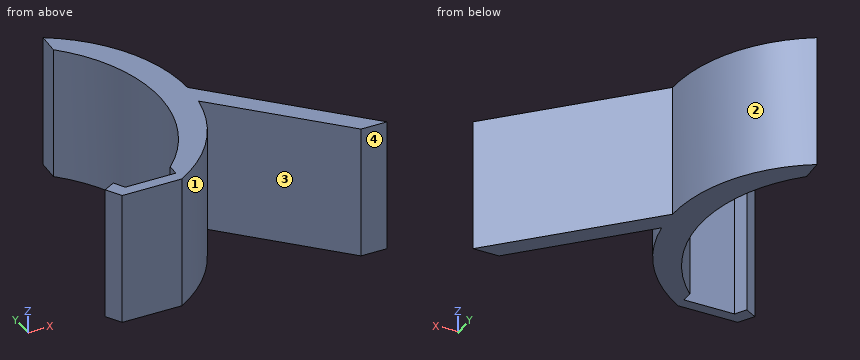
```python
from build123d import *

# Parameters (mm, degrees)
F1_DEPTH = 76.2


with BuildPart() as f1:
    # F0 (on Top) → F1 (new body)
    with BuildSketch(Plane.XY):
        Polygon((-34.220355, 0), (-25.4, 0), (-29.066174, 6.35), (-32.732348, 12.7), (-39.347615, 8.880674), align=None)
        with BuildLine():
            Line((-25.4, 0), (0, 0))
            ThreePointArc((0, 0), (27.857567, 26.408715), (41.984283, 62.100452))
            ThreePointArc((41.984283, 62.100452), (42.827748, 69.127812), (43.109499, 76.2))
            ThreePointArc((43.109499, 76.2), (31.585159, 119.974618), (0, 152.4))
            Line((0, 152.4), (-0.635, 139.7))
            ThreePointArc((-0.635, 139.7), (26.365937, 76.333417), (0, 12.7))
            Line((0, 12.7), (0, 6.35))
            Line((0, 6.35), (-29.066174, 6.35))
            Line((-29.066174, 6.35), (-25.4, 0))
        make_face()
        with BuildLine():
            ThreePointArc((43.109499, 76.2), (42.827748, 69.127812), (41.984283, 62.100452))
            Line((41.984283, 62.100452), (102.847256, 0))
            Line((102.847256, 0), (117.791057, 0))
            Line((117.791057, 0), (43.109499, 76.2))
        make_face()
    extrude(amount=F1_DEPTH)


solid = f1.part
```
Here's how the part is built. I have some questions about the finished solid (model axes, mm). Face numbers are marked on the shaded views. Coordinates: 2 decimals unless noted, no trailing zeros. Write each loop counter-clockwise with the first axis right and the second up, starting at its lowest first coordinate (ties: lowest second). Pieces come first, ordered by that corner, then holes. Notation, with made-up numbers: (88.5, 72) -> (138.5, 72) arc R31 ccw to (138.5, 102) -> close; hole circle Ø8 at (65.25, -25.5). An arc over 180 degrees is marked (long way). Use a Markdown table: item, result. Add a question column.
(1) We'd pull the mould along X, two halves only. Please class the marked faces 1, 2, 3 and 4: +X half, -X half, draft (parallel to the pull), parting line (faces both ways), or undercut.
(2) If we section it at D-D, the plane x = -20.5: Write out the boundary of the cut face in (y, z), and give its area (3 significant figures).
(3) I'm going to push flat-ended pins straight in: P1, Ø14.5, axis at x = -20.5, z = 48.5, coming from the +Y side; P2, Ø4, axis at y = 136.5, z = 45.5, coming from the -X side; P3, Ø10, axis at y = 75, z = 33.5, coming from the -X side. Where does each tip first touch, or does it pass through?
(4) If we section it at B-B, the plane y = 24.5: Write out the boundary of the cut face in (x, z).
(5) If we section it at C-C, the plane x = 22.5: Write out the boundary of the cut face in (y, z), and give its area (3 significant figures).
(6) Please list where these lines run through material, in increasing order: line 1 (X direction, y = 12.5, z = 72); line 2 (Y direction, x = -9, z = 60); line 3 (X direction, y = 17.5, z = 10.5).
Outcome:
| question | item | result |
|---|---|---|
| 1 | face 1 | undercut |
| 1 | face 2 | +X half |
| 1 | face 3 | undercut |
| 1 | face 4 | draft |
| 2 | outline | (0, 0) -> (6.35, 0) -> (6.35, 76.2) -> (0, 76.2) -> close |
| 2 | area | 484 mm^2 |
| 3 | P1 | stops at y = 6.35 |
| 3 | P2 | stops at x = 0.58 |
| 3 | P3 | stops at x = 26.17 |
| 4 | outline | (10.01, 0) -> (26.53, 0) -> (26.53, 76.2) -> (10.01, 76.2) -> close; (78.84, 0) -> (93.78, 0) -> (93.78, 76.2) -> (78.84, 76.2) -> close |
| 5 | outline | (19.28, 0) -> (49.95, 0) -> (49.95, 76.2) -> (19.28, 76.2) -> close; (101.82, 0) -> (133.12, 0) -> (133.12, 76.2) -> (101.82, 76.2) -> close |
| 5 | area | 4,720 mm^2 |
| 6 | line 1 | x = -33.08 to -32.62, 0 to 16.22, 90.6 to 105.54 |
| 6 | line 2 | y = 0 to 6.35 |
| 6 | line 3 | x = 4.5 to 20.97, 85.7 to 100.64 |
